from build123d import *

# Parameters (mm, degrees)
EXTRUDE_2_DEPTH          = 60
CUT_EXTRUDE_2_DEPTH      = 76.498344353
CUT_EXTRUDE_2_DEPTH_BACK = 76.498344353


with BuildPart() as part:
    # Sketch 1 → Extrude 2 (new body)
    with BuildSketch(Plane(origin=(0, 0, 0), x_dir=(0, 0, -1), z_dir=(1, 0, 0))):
        Polygon((30, -17.320508076), (30, 17.320508076), (0, 34.641016151), (-30, 17.320508076), (-30, -17.320508076), (0, -34.641016151), align=None)
        Polygon((30, 34.641016151), (0, 34.641016151), (30, 17.320508076), align=None)
        Polygon((-30, 34.641016151), (-30, 17.320508076), (0, 34.641016151), align=None)
    extrude(amount=EXTRUDE_2_DEPTH)

    # Sketch 3 → Cut-Extrude 2 (cut, two sides: drawn at the far end of the back side and taken through both)
    with BuildSketch(Plane.XY.offset(-CUT_EXTRUDE_2_DEPTH_BACK)):
        Polygon((60, 0), (30, 0), (0, 34.641016151), (60, 34.641016151), align=None)
    extrude(amount=CUT_EXTRUDE_2_DEPTH + CUT_EXTRUDE_2_DEPTH_BACK, mode=Mode.SUBTRACT)


solid = part.part
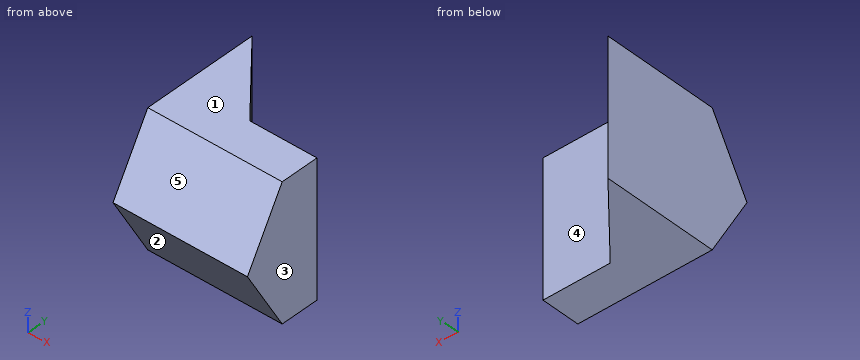
The listing builds one solid part. Answer for the finished solid, in the listing's coordinates (mm). Face numbers are marked on the shaded views. A direction names the side the tool comes from. Round coordinates to 2 decimals unless told otherwise and drop trailing zeros. Write each loop counter-clockwise with the first axis right and the second up, starting at its lowest first coordinate (ties: lowest second). Pieces come first, ordered by that corner, then holes. Notation, with made-up numbers: (24, 67) - (63, 67) arc R26 ccw to (63, 84) - close; hole circle Ø5 at (68, 37). An arc over 180 degrees is marked (long way). Use one line per item in the form item = value. Start each with the question number.
Item 1: A cutting plane is placed at D-D (y = 11.5). Write down the section's boundary in (x, z).
Item 2: Find the intervals of material crossed by line 1 (Y direction, x = 56.5, z = 0); line 2 (X direction, y = 15, z = -13.5); line 3 (Z direction, x = 5.5, y = -20.5), in increasing order. Write a range as [from, to].
Item 3: Flat-ended cylindrical pins translate along their axes: pin 1 Ø10 at (y, z) = (12.5, -7.5) entering from +X; pin 2 Ø1 at (x, z) = (15.5, -9) entering from +Y; pin 3 Ø8 at (y, z) = (27, -17.5) entering from +X. Find the tip coordinate at first contact, or state that the pin passes through.
Item 4: A cutting plane is placed at A-A (x = 46). Write down the section's boundary in (y, z), plus the area to 3 significant figures.
Item 5: A cutting plane is placed at C-C (y = -25). Write down the section's boundary in (x, z).
Item 6: A cutting plane is placed at B-B (z = 15). Write down the section's boundary in (x, y).
Item 7: A tool of negligible diameter and unlimited length cuts with its end or side. For the marked faces 4 and 5, from which of +Z, -Z, +X, -X, +Y, -Y can it reach the whole face along a straight path? Write none if from no direction.
Item 8: Determine the mould class of the marked faces 1, 2 and 3 for opening direction Z: +Z half, -Z half, draft (parallel to the pull), parting line (faces both ways), or undercut.
The answers:
q1.outline = (0, -30) - (20.04, -30) - (20.04, 30) - (0, 30) - close
q2.line_1 = [-34.64, 0]
q2.line_2 = [0, 17.01]
q2.line_3 = [-24.49, 24.49]
q3.pin_1 = 23.5
q3.pin_2 = 17.32
q3.pin_3 = 10.08
q4.outline = (-34.64, 0) - (-17.32, -30) - (0, -30) - (0, 30) - (-17.32, 30) - close
q4.area = 1,560 mm^2
q5.outline = (0, -16.7) - (60, -16.7) - (60, 16.7) - (0, 16.7) - close
q6.outline = (0, -25.98) - (60, -25.98) - (60, 0) - (30, 0) - (0, 34.64) - close
q7.face_4 = +Z, -Z, +X, +Y
q7.face_5 = +Z, +X, -X, -Y
q8.face_1 = +Z half
q8.face_2 = -Z half
q8.face_3 = draft
